Geometry check sheet. Reference: the model listing, model coordinates, mm. A direction names the side the tool comes from. Round coordinates to 2 decimals unless told otherwise and drop trailing zeros. Loops run counter-clockwise (first coordinate to the right, second up) from the corner with the lowest first, then second, coordinate; pieces in that order, holes last.
Autodesk Inventor part; units mm, degrees
ref_plane "YZ Plane" through (0, 0, 0) normal (1, 0, 0) x (0, 1, 0)
ref_plane "XZ Plane" through (0, 0, 0) normal (0, 1, 0) x (-1, 0, 0)
ref_plane "XY Plane" through (0, 0, 0) normal (0, 0, 1) x (1, 0, 0)
sketch "Sketch_18" plane through (0, 0, 0) normal (0, 0, 1) x (1, 0, 0)
  line L0 (50, 0) -> (-50, 0)
  arc A0 (0, 1.6) -> (0.1, 1.5) centre (0.1, 1.6) ccw
  line L1 (0.1, 1.5) -> (2.9, 1.5)
  arc A1 (2.9, 1.5) -> (3, 1.6) centre (2.9, 1.6) ccw
  line L2 (3, 1.6) -> (3, 2.5)
  line L3 (3, 2.5) -> (1.8969, 2.5)
  arc A2 (1.1031, 2.5) -> (1.8969, 2.5) centre (1.5, 2.95) ccw
  line L4 (1.1031, 2.5) -> (0, 2.5)
  line L5 (0, 2.5) -> (0, 1.6)
revolve "Revolution1" add sketch "Sketch_18" angle 360 about axis through (50, 0, 0) along (1, 0, 0)
sketch "Sketch_20" plane through (0, 0, 0) normal (0, 0, 1) x (1, 0, 0)
  line L0 (50, 0) -> (-50, 0)
  line L1 (0.09, 3.7) -> (0.105, 3.3975)
  line L2 (0.105, 3.3975) -> (0.09, 3.095)
  line L3 (0.09, 3.095) -> (0.09, 2.49)
  line L4 (0.09, 2.49) -> (0.12, 2.49)
  line L5 (0.12, 2.49) -> (0.15, 3.095)
  line L6 (0.15, 3.095) -> (0.15, 3.3975)
  line L7 (0.15, 3.3975) -> (0.12, 3.7)
  line L8 (0.12, 3.7) -> (0.09, 3.7)
revolve "Revolution2" add sketch "Sketch_20" angle 360 about axis through (50, 0, 0) along (1, 0, 0)
sketch "Sketch_21" plane through (0, 0, 0) normal (0, 0, 1) x (1, 0, 0)
  line L0 (50, 0) -> (-50, 0)
  line L1 (2.85, 3.3975) -> (2.85, 3.095)
  line L2 (2.85, 3.095) -> (2.88, 2.49)
  line L3 (2.88, 2.49) -> (2.91, 2.49)
  line L4 (2.91, 2.49) -> (2.91, 3.095)
  line L5 (2.91, 3.095) -> (2.895, 3.3975)
  line L6 (2.895, 3.3975) -> (2.91, 3.7)
  line L7 (2.91, 3.7) -> (2.88, 3.7)
  line L8 (2.88, 3.7) -> (2.85, 3.3975)
revolve "Revolution3" add sketch "Sketch_21" angle 360 about axis through (50, 0, 0) along (1, 0, 0)
properties part number "SKF_W 619/3-2Z_PART1"
1) Access from +Z, -Z, +X, -X, +Y, -Y to the whole of each face (thin tool, end or side, straight path). Record for faces 3 (the face through (0, 2, 0)), 4 (the face through (2.38, -0.54, 2.44)).
Report:
face 3: +Z, -Z, -X, +Y, -Y
face 4: none
2) Scan lines: line 1 along Z through (x, y) = (1.95, 0); line 2 along Z through (x, y) = (0.5, 2). Record each from-to range of solid material in increasing order.
Report:
line 1: z = -2.5 to -1.5, 1.5 to 2.5
line 2: z = -1.5 to 1.5
3) Mould release check, pull along Y, two halves, no side actions. Record for faces 1 (the face through (3, 2, 0)), 2 (the face through (1.52, -1.5, 0.07)): +Y half, -Y half, draft (parallel to the pull), parting line (faces both ways), or undercut.
Report:
face 1: draft
face 2: undercut
4) Sectioned sample at A-A, the plane x = 0.25. Record the cut outline in (y, z), then the cut area to 3 significant figures.
Report:
outline: circle Ø5 at (0, 0); hole circle Ø3 at (0, 0)
area: 12.6 mm2
5) Gauge pin test, flat ends, axial feed: pin 1 (1.5 mm diameter, centred on y = 1, z = 1.5, fed in from -X); pin 2 (1.5 mm diameter, centred on y = 2.5, z = 2.5, fed in from +X); pin 3 (1 mm diameter, centred on x = 2, z = -2, fed in from -Y); pin 4 (1.5 mm diameter, centred on x = 1.5, y = -2.5, fed in from -Z). Record the tip position at first contact, or that the pin passes through.
Report:
pin 1: stops at x = 0
pin 2: stops at x = 2.91
pin 3: stops at y = -2
pin 4: stops at z = -1.67
